Autodesk Fusion 360 part; units mm, degrees
sketch "Boceto1" plane through (0, 0, 0) normal (0, 1, 0) x (1, 0, 0)
  line L0 (2.05, 0) -> (0, 0) construction
  line L1 (3.05, 0) -> (15.65, 0)
  line L2 (2.05, -12.3964) -> (2.05, -1)
  arc A0 (3.05, 0) -> (2.05, -1) centre (3.05, -1) ccw
  line L3 (3.6762, -10.8738) -> (3.6762, -1.8762)
  line L4 (3.9262, -1.6262) -> (15.65, -1.6262)
  arc A1 (3.9262, -1.6262) -> (3.6762, -1.8762) centre (3.9262, -1.8762) ccw
  line L5 (1.9767, -12.5732) -> (-0.0927, -14.6402)
  line L6 (0.5221, -15.8217) -> (-0.093, -15.2059)
  arc A2 (-0.0927, -14.6402) -> (-0.093, -15.2059) centre (0.19, -14.9232) ccw
  line L7 (0.8, -16.4931) -> (0.8, -18.25)
  line L8 (0.6, -18.45) -> (0.45, -18.45)
  arc A3 (0.8, -16.4931) -> (0.5221, -15.8217) centre (-0.15, -16.4931) ccw
  arc A4 (0.6, -18.45) -> (0.8, -18.25) centre (0.6, -18.25) ccw
  line L9 (3.6762, -10.8738) -> (3.6762, -13.0203)
  line L10 (2.5, -14.3) -> (3.6029, -13.1971)
  line L11 (2.5, -14.3) -> (2.5, -18.0672)
  line L12 (2.7322, -18.3166) -> (5.0322, -18.4809)
  line L13 (5.3, -18.2315) -> (5.3, -17.95)
  line L14 (5.9, -17.35) -> (6.35, -17.35)
  line L15 (6.95, -17.95) -> (6.95, -19.5)
  line L16 (6.35, -20.1) -> (5.3, -20.1)
  line L17 (-0.1, -19) -> (-0.1, -19.0559)
  arc A5 (0.3391, -19.5946) -> (5.3, -20.1) centre (5.3, 4.5) ccw
  arc A6 (-0.1, -19.0559) -> (0.3391, -19.5946) centre (0.45, -19.0559) ccw
  arc A7 (0.45, -18.45) -> (-0.1, -19) centre (0.45, -19) ccw
  arc A8 (6.35, -20.1) -> (6.95, -19.5) centre (6.35, -19.5) ccw
  arc A9 (6.95, -17.95) -> (6.35, -17.35) centre (6.35, -17.95) ccw
  arc A10 (5.9, -17.35) -> (5.3, -17.95) centre (5.9, -17.95) ccw
  arc A11 (5.0322, -18.4809) -> (5.3, -18.2315) centre (5.05, -18.2315) ccw
  arc A12 (2.5, -18.0672) -> (2.7322, -18.3166) centre (2.75, -18.0672) ccw
  arc A13 (3.6029, -13.1971) -> (3.6762, -13.0203) centre (3.4262, -13.0203) ccw
  arc A14 (1.9767, -12.5732) -> (2.05, -12.3964) centre (1.8, -12.3964) ccw
  line L18 (15.65, 0) -> (15.65, -24.4844) construction
  line L19 (28.8, -14.3) -> (27.6971, -13.1971)
  line L20 (27.6238, -10.8738) -> (27.6238, -13.0203)
  arc A15 (24.35, -19.5) -> (24.95, -20.1) centre (24.95, -19.5) ccw
  line L21 (30.7, -18.45) -> (30.85, -18.45)
  line L22 (29.25, -12.3964) -> (29.25, -1)
  line L23 (26, -18.2315) -> (26, -17.95)
  line L24 (28.8, -14.3) -> (28.8, -18.0672)
  line L25 (30.7779, -15.8217) -> (31.393, -15.2059)
  arc A16 (30.5, -18.25) -> (30.7, -18.45) centre (30.7, -18.25) ccw
  line L26 (31.4, -19) -> (31.4, -19.0559)
  arc A17 (31.4, -19) -> (30.85, -18.45) centre (30.85, -19) ccw
  arc A18 (29.25, -1) -> (28.25, 0) centre (28.25, -1) ccw
  arc A19 (31.393, -15.2059) -> (31.3927, -14.6402) centre (31.11, -14.9232) ccw
  line L27 (25.4, -17.35) -> (24.95, -17.35)
  line L28 (29.3233, -12.5732) -> (31.3927, -14.6402)
  arc A20 (24.95, -17.35) -> (24.35, -17.95) centre (24.95, -17.95) ccw
  arc A21 (29.25, -12.3964) -> (29.3233, -12.5732) centre (29.5, -12.3964) ccw
  arc A22 (30.9609, -19.5946) -> (31.4, -19.0559) centre (30.85, -19.0559) ccw
  arc A23 (26, -18.2315) -> (26.2678, -18.4809) centre (26.25, -18.2315) ccw
  line L29 (29.25, 0) -> (31.3, 0) construction
  arc A24 (26, -20.1) -> (30.9609, -19.5946) centre (26, 4.5) ccw
  line L30 (24.35, -17.95) -> (24.35, -19.5)
  line L31 (24.95, -20.1) -> (26, -20.1)
  arc A25 (27.6238, -1.8762) -> (27.3738, -1.6262) centre (27.3738, -1.8762) ccw
  arc A26 (26, -17.95) -> (25.4, -17.35) centre (25.4, -17.95) ccw
  line L32 (30.5, -16.4931) -> (30.5, -18.25)
  arc A27 (28.5678, -18.3166) -> (28.8, -18.0672) centre (28.55, -18.0672) ccw
  line L33 (28.5678, -18.3166) -> (26.2678, -18.4809)
  line L34 (27.6238, -10.8738) -> (27.6238, -1.8762)
  arc A28 (30.7779, -15.8217) -> (30.5, -16.4931) centre (31.45, -16.4931) ccw
  arc A29 (27.6238, -13.0203) -> (27.6971, -13.1971) centre (27.8738, -13.0203) ccw
  line L35 (27.3738, -1.6262) -> (15.65, -1.6262)
  line L36 (28.25, 0) -> (15.65, 0)
  point P0 (31.3, 0)
  dimension "d1" = 1
  dimension "d3" = 0.25
  dimension "d4" = 0.4
  dimension "d5" = 0.95
  dimension "d6" = 0.2
  dimension "d7" = 0.55
  dimension "d8" = 0.6
  dimension "d9" = 0.25
extrude "Extruir1" add sketch "Boceto1" along normal blind 10
Part model, mm, in its own coordinate system. A direction names the side the tool comes from. Round coordinates to 2 decimals unless told otherwise and drop trailing zeros. Loops run counter-clockwise (first coordinate to the right, second up) from the corner with the lowest first, then second, coordinate; pieces in that order, holes last.
1. Slice it at C-C (x = 8). Give the cut face in (y, z).
Solutions:
outline: (0, 0) - (10, 0) - (10, 1.63) - (0, 1.63) - close
2. Two-plate mould, pull along Z, no slides. Class faces 1 (the face through (24.35, 5, 19)), 2 (the face through (30.5, 5, 17)), 3 (the face through (2.841, 4.93, 19.977)): pulls with the +Z half, pulls with the -Z half, needs draft (parallel to the pull), parting line crosses it, or undercut.
Solutions:
face 1: needs draft
face 2: undercut
face 3: pulls with the +Z half
3. Drill centre lines: line 1 along Z through (x, y) = (25, 4.75); line 2 along X through (y, z) = (2.75, 17.25); line 3 along X through (y, z) = (4.5, 4). Where is each one in solid material? Low to high.
Solutions:
line 1: z = 0 to 1.63, 17.35 to 20.1
line 2: x = 0.8 to 2.5, 28.8 to 30.5
line 3: x = 2.05 to 3.68, 27.62 to 29.25
4. Flat gauge pins, fed straight in: pin 1 (5 mm diameter, centred on y = 8.5, z = 6.5, fed in from -X); pin 2 (1.7 mm diameter, centred on y = 7, z = 18.5, fed in from -X); pin 3 (3 mm diameter, centred on y = 7.5, z = 5.5, fed in from +X); pin 4 (12 mm diameter, centred on x = 18.5, z = 18, fed in from -Y). Where does each tip first touch, or does it go through?
Solutions:
pin 1: stops at x = 2.05
pin 2: stops at x = -0.1
pin 3: stops at x = 29.25
pin 4: stops at y = 0
5. 3-axis set-ups, long thin cutter, end or side, ignore diameter. For faces 4 (the face through (29.25, 5, 7)), 5 (the face through (0.8, 5, 17)), 6 (the face through (2.05, 5, 7)), 7 (the face through (16, 5, 1.626)): which of +Z, -Z, +X, -X, +Y, -Y reach the whole face in a straight line?
Solutions:
face 4: -Z, +X, +Y, -Y
face 5: -X, +Y, -Y
face 6: -Z, -X, +Y, -Y
face 7: +Y, -Y
6. Slice it at A-A (z = 17). Give the cut face in (x, y), and give its area (3 significant figures).
Solutions:
outline: (0.8, 0) - (2.5, 0) - (2.5, 10) - (0.8, 10) - close; (28.8, 0) - (30.5, 0) - (30.5, 10) - (28.8, 10) - close
area: 34.0 mm2
7. Slice it at B-B (z = 5.75). Give the cut face in (x, y).
Solutions:
outline: (2.05, 0) - (3.68, 0) - (3.68, 10) - (2.05, 10) - close; (27.62, 0) - (29.25, 0) - (29.25, 10) - (27.62, 10) - close
